```python
from build123d import *

# Parameters (mm, degrees)
SKETCH1_W               = 38.1
SKETCH1_H               = 38.1
SKETCH1_W_2             = 31.75
SKETCH1_H_2             = 31.75
BOSS_EXTRUDE1_DEPTH     = 230.1875
FILLET1_R               = 3.81
FILLET2_R               = 0.635
SKETCH2_R               = 3.175
CUT_EXTRUDE1_DEPTH      = 20.05
CUT_EXTRUDE1_DEPTH_BACK = 20.05


with BuildPart() as part:
    # Sketch1 → Boss-Extrude1 (new body, symmetric)
    with BuildSketch(Plane.XY):
        Rectangle(SKETCH1_W, SKETCH1_H)
        Rectangle(SKETCH1_W_2, SKETCH1_H_2, mode=Mode.SUBTRACT)
    extrude(amount=BOSS_EXTRUDE1_DEPTH, both=True)

    # Fillet1
    fillet1_edges = [part.edges().sort_by_distance(p)[0] for p in [
        (19.05, -19.05, 0),
        (-19.05, -19.05, 0),
        (-19.05, 19.05, 0),
        (19.05, 19.05, 0),
    ]]
    fillet(fillet1_edges, radius=FILLET1_R)

    # Fillet2
    fillet2_edges = [part.edges().sort_by_distance(p)[0] for p in [
        (15.875, 15.875, 0),
        (-15.875, 15.875, 0),
        (-15.875, -15.875, 0),
        (15.875, -15.875, 0),
    ]]
    fillet(fillet2_edges, radius=FILLET2_R)

    # Sketch2 → Cut-Extrude1 (cut, two sides)
    with BuildSketch(Plane(origin=(0, 0, 0), x_dir=(1, 0, 0), z_dir=(0, 1, 0))) as cut_extrude1_sk:
        with Locations((0, -211.1375)):
            Circle(SKETCH2_R)
        with Locations((0, -102.4)):
            Circle(SKETCH2_R)
        with Locations((0, -37.4)):
            Circle(SKETCH2_R)
        with Locations((0, 37.4)):
            Circle(SKETCH2_R)
        with Locations((0, 102.4)):
            Circle(SKETCH2_R)
        with Locations((0, 211.1375)):
            Circle(SKETCH2_R)
    extrude(amount=CUT_EXTRUDE1_DEPTH, mode=Mode.SUBTRACT)
    extrude(cut_extrude1_sk.sketch, amount=-CUT_EXTRUDE1_DEPTH_BACK, mode=Mode.SUBTRACT)


solid = part.part
```
Input: part model. Units: mm. Frame: model coordinates. A direction names the side the tool comes from. Round coordinates to 2 decimals unless told otherwise and drop trailing zeros. Write each loop counter-clockwise with the first axis right and the second up, starting at its lowest first coordinate (ties: lowest second). Pieces come first, ordered by that corner, then holes. Notation, with made-up numbers: (-33, 67.25) - (4, 67.25) arc R32 cw to (4, 100.25) - close; hole circle Ø1 at (9, -12). An arc over 180 degrees is marked (long way). Write item = value, one per line.
(1) Material intervals for probe 1 along Y at (x, z) = (-5, -171.5) (3 decimals); probe 2 along X at (y, z) = (-17, -102), sorted ascending.
Geometry check:
probe_1 = -19.05 to -15.875, 15.875 to 19.05
probe_2 = -18.62 to -3.15, 3.15 to 18.62
(2) Pull-direction query (Y, two-part tool) for faces 1 (the flat face through (-19.05, 0, 3)), 2 (the flat face through (0, -15.875, 3)), 3 (the flat face through (0, 19.05, 3)), 4 (the flat face through (0, -19.05, 3)); classes: +Y half, -Y half, draft (parallel to the pull), parting line (faces both ways), or undercut.
Geometry check:
face_1 = draft
face_2 = undercut
face_3 = +Y half
face_4 = -Y half
(3) Contact query for a flat-ended pin moving along its axis: pin 1 Ø5 at (x, z) = (0, -37.4) entering from +Y. Output: stop coordinate, or through.
Geometry check:
pin_1 = through
(4) Section query B-B on z = -159.5. Output: boundary loops of the cut face in (x, y) (3 decimals).
Geometry check:
outline = (-19.05, -15.24) arc R3.81 ccw to (-15.24, -19.05) - (15.24, -19.05) arc R3.81 ccw to (19.05, -15.24) - (19.05, 15.24) arc R3.81 ccw to (15.24, 19.05) - (-15.24, 19.05) arc R3.81 ccw to (-19.05, 15.24) - close; hole (-15.875, -15.24) arc R0.635 ccw to (-15.24, -15.875) - (15.24, -15.875) arc R0.635 ccw to (15.875, -15.24) - (15.875, 15.24) arc R0.635 ccw to (15.24, 15.875) - (-15.24, 15.875) arc R0.635 ccw to (-15.875, 15.24) - close
(5) Access query for faces 5 (the flat face through (0, 15.875, 3)), 6 (the flat face through (-17, 0, 230.188)). Directions: +Z, -Z, +X, -X, +Y, -Y. A direction counts if a zero-diameter tool reaches every point of the face in a straight line with its end or side. Return the directions, or none.
Geometry check:
face_5 = +Z, -Z
face_6 = +Z, +X, -X, +Y, -Y
